Geometry check sheet. Reference: drawing and pictorial views, mm from the part's lowest x, y, z. A direction names the side the tool comes from. Round coordinates to 2 decimals unless told otherwise and drop trailing zeros. Write each loop counter-clockwise with the first axis right and the second up, starting at its lowest first coordinate (ties: lowest second). Pieces come first, ordered by that corner, then holes. Notation, with made-up numbers: (85.5, 2) -> (135.5, 2) arc R5 ccw to (135.5, 10) -> close; hole circle Ø7 at (29.25, 40.25). An arc over 180 degrees is marked (long way). Answer as a JSON object with one key per item and string values. Group by question number.
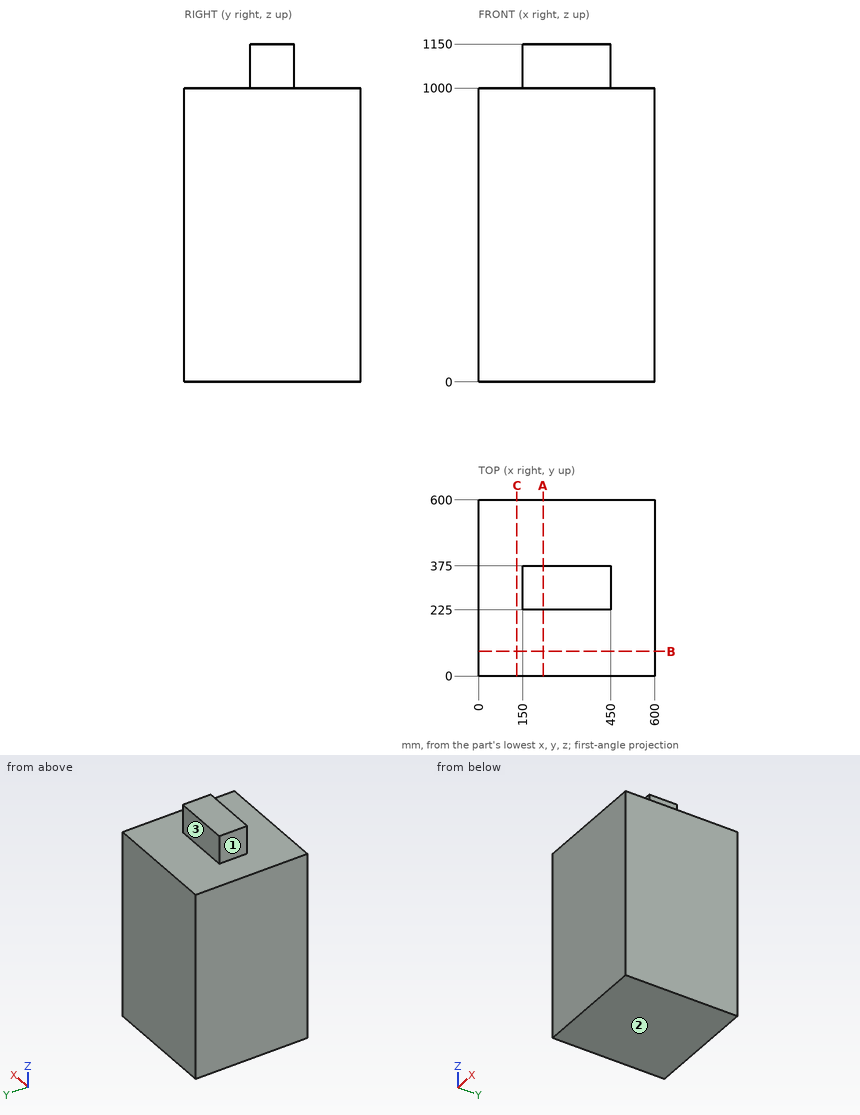
(1) Scan lines: line 1 along Y through (x, z) = (246, 1010); line 2 along Z through (x, y) = (271.5, 211). Record each from-to range of solid material in increasing order.
(2) Go/stop test with a flat-tipped pin: pin 1 Ø8 at (x, y) = (106.5, 88) entering from +Z. Record where the tip stops, or that it passes through.
(3) Section check B-B on y = 83.5. Record the cut outline in (x, z).
(4) Access from +Z, -Z, +X, -X, +Y, -Y to the whole of each face (thin tool, end or side, straight path). Record for the marked faces 1, 2 and 3.
(5) Section check A-A on x = 220. Record the cut outline in (y, z).
Data:
{
 "1": {"line 1": "y = 225 to 375", "line 2": "z = 0 to 1000"},
 "2": {"pin 1": "stops at z = 1000"},
 "3": {"outline": "(0, 0) -> (600, 0) -> (600, 1000) -> (0, 1000) -> close"},
 "4": {"face 1": "+Z, -X, +Y, -Y", "face 2": "-Z, +X, -X, +Y, -Y", "face 3": "+Z, +X, -X, +Y"},
 "5": {"outline": "(0, 0) -> (600, 0) -> (600, 1000) -> (375, 1000) -> (375, 1150) -> (225, 1150) -> (225, 1000) -> (0, 1000) -> close"}
}
